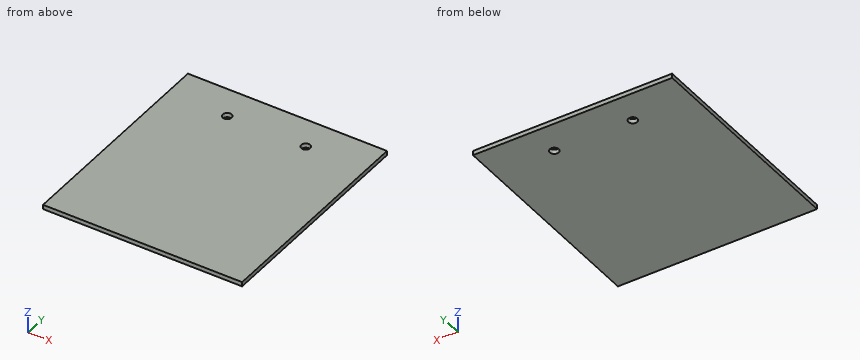
Autodesk Fusion 360 part; units mm, degrees
sketch "Sketch1" plane through (0, 0, 0) normal (0, 0, 1) x (1, 0, 0)
  line L0 (0, 0) -> (90, 0)
  line L1 (90, 0) -> (90, 100)
  line L2 (90, 100) -> (0, 100)
  line L3 (0, 100) -> (0, 0)
  line L4 (45, 100) -> (45, 0)
  line L5 (90, 50) -> (0, 50)
  line L6 (45, 85.5) -> (49, 85.5) construction
  circle A0 centre (45, 85.5) radius 3 construction
  line L7 (45, 85.5) -> (27.25, 85.5) construction
  line L8 (45, 85.5) -> (62.75, 85.5) construction
  circle A1 centre (27.25, 85.5) radius 2
  circle A2 centre (62.75, 85.5) radius 2
  dimension "d1" = 90
  dimension "d2" = 100
  dimension "d3" = 14.5
  dimension "d4" = 6
  dimension "d5" = 17.75
  dimension "d6" = 4
extrude "Extrude1" add sketch "Sketch1" along normal blind 2
Verification items for the finished model (mm, model axes). Give positions to 0.01 mm unless a question says otherwise; leave off trailing zeros. Order: outer loops, then holes, each group sorted by start corner. A loop starts at its lowest first (then second) coordinate and runs counter-clockwise, first axis right, second up. Notation, with made-up numbers: M -23,89.5 L 27,89.5 A28 cw 27,118.5 Z; hole C 33,16.5 d4. An arc over 180 degrees is marked long. Answer in a Markdown table with one row per item. Add a question column.
Item 1: Section check B-B, the plane x = 27.25. Enter the section's corners in (y, z).
Item 2: Gauge pin test, flat end, axial feed: pin 1 (4 mm diameter, centred on x = 13.5, y = 77.5, fed in from -Z). Record the tip position at first contact, or that the pin passes through.
Item 3: Section check A-A, the plane y = 85.5. Enter the section's corners in (x, z), and give its area (3 significant figures).
Item 4: Scan lines: probe 1 along Y at (x, z) = (27.25, 1.5); probe 2 along Y at (x, z) = (61.5, 1.8). Record each from-to range of solid material in increasing order. Write a range as from..to.
Filled sheet:
| question | item | result |
|---|---|---|
| 1 | outline | M 0,0 L 83.5,0 L 83.5,2 L 0,2 Z; M 87.5,0 L 100,0 L 100,2 L 87.5,2 Z |
| 2 | pin 1 | stops at z = 0 |
| 3 | outline | M 0,0 L 25.25,0 L 25.25,2 L 0,2 Z; M 29.25,0 L 60.75,0 L 60.75,2 L 29.25,2 Z; M 64.75,0 L 90,0 L 90,2 L 64.75,2 Z |
| 3 | area | 164 mm^2 |
| 4 | probe 1 | y = 0..83.5, 87.5..100 |
| 4 | probe 2 | y = 0..83.94, 87.06..100 |
